from build123d import *

# Parameters (mm, degrees)
CUT_EXTRUDE1_DEPTH = 1


with BuildPart() as part:
    # Sketch1 → Revolve1 (revolve)
    with BuildSketch(Plane.XY, mode=Mode.PRIVATE) as revolve1_sk:
        with BuildLine():
            Line((0, 0), (0, 1.425))
            ThreePointArc((0, 1.425), (0.342509352, 2.900635456), (1.3, 4.07452826))
            Line((1.3, 4.07452826), (1.65, 4.07452826))
            Line((1.65, 4.07452826), (1.65, 1.5))
            Line((1.65, 1.5), (38.35, 1.5))
            Line((38.35, 1.5), (38.65, 1.2))
            Line((38.65, 1.2), (38.65, 0))
            Line((38.65, 0), (0, 0))
        make_face()
    revolve(revolve1_sk.sketch.rotate(Axis((0, 0, 0), (1, 0, 0)), 90), axis=Axis((0, 0, 0), (1, 0, 0)))

    # Sketch2 → Cut-Extrude1 (cut)
    with BuildSketch(Plane.ZY):
        Polygon((0, 1.154700538), (-1, 0.577350269), (-1, -0.577350269), (0, -1.154700538), (1, -0.577350269), (1, 0.577350269), align=None)
    extrude(amount=-CUT_EXTRUDE1_DEPTH, mode=Mode.SUBTRACT)


solid = part.part
Work out the finished part from the listing and answer in its coordinate system (mm). A direction names the side the tool comes from. Give positions to 0.01 mm unless a question says otherwise; leave off trailing zeros. Write each loop counter-clockwise with the first axis right and the second up, starting at its lowest first coordinate (ties: lowest second). Pieces come first, ordered by that corner, then holes. Notation, with made-up numbers: (70.5, 19.5) - (126.5, 19.5) arc R21 ccw to (126.5, 44.5) - close; hole circle Ø8 at (40, 12). An arc over 180 degrees is marked (long way). One line per item, written item: value. Start each with the question number.
1. Find section A-A (x = 22). Write down the section's boundary in (y, z).
2. For a pull along Y with two mould halves and no side action, classify faces 4 (the cylindrical face through (1.477, -1.224, 3.886)), 5 (the flat face through (0.5, 0, -1)), 6 (the flat face through (1.65, 0, 2)) as +Y half, -Y half, draft (parallel to the pull), parting line (faces both ways), or undercut.
3. Given pin 1 (4 mm diameter, centred on x = 12, z = -3, fed in from +Y); pin 2 (2 mm diameter, centred on y = -2.5, z = 0.5, fed in from +X); pin 3 (3 mm diameter, centred on x = 13, z = -1.5, fed in from +Y), each flat-ended and moving along its own axis, determine where each tip first touches the part or whether it passes through.
4. For faces 1 (the flat face through (0.49, 0.86, 0.51)), 2 (the cylindrical face through (20.26, -0.45, 1.43)), 3 (the flat face through (38.65, 0, 0)), determine the directions among +Z, -Z, +X, -X, +Y, -Y from which every point of the face is accessible in a straight line to the end or side of a thin tool.
5. Consider probe 1 along Y at (x, z) = (36, 0); probe 2 along X at (y, z) = (0.75, -0.5); probe 3 along X at (y, z) = (1.75, -0.5). Determine where each line is inside the solid, lowest interval first.
Geometry results:
1. outline: circle Ø3 at (0, 0)
2. face 4: parting line
2. face 5: undercut
2. face 6: draft
3. pin 1: y = 1.12
3. pin 2: x = 1.65
3. pin 3: y = 1.5
4. face 1: -X
4. face 2: +X
4. face 3: +Z, -Z, +X, +Y, -Y
5. probe 1: -1.5 to 1.5
5. probe 2: 1 to 38.65
5. probe 3: 0.02 to 1.65
